Work out the finished part from the listing and answer in its coordinate system (mm). Face numbers are marked on the shaded views. A direction names the side the tool comes from. Give positions to 0.01 mm unless a question says otherwise; leave off trailing zeros. Write each loop counter-clockwise with the first axis right and the second up, starting at its lowest first coordinate (ties: lowest second). Pieces come first, ordered by that corner, then holes. Notation, with made-up numbers: (55, -29.5) -> (110, -29.5) arc R16 cw to (110, -14.5) -> close; hole circle Ø11 at (66.5, 50.25). An arc over 180 degrees is marked (long way). Use a Markdown table: item, result. Add a question column.
Q1. Consider line 1 (Y direction, x = 53.5, z = 1.1); line 2 (Z direction, x = 38.7, y = 46.25); line 3 (X direction, y = 49.5, z = 0.5). Determine where each line is inside the solid, lowest interval first.
Q2. Section C-C, the plane x = 38.7 is taken. Give the vertices of the cut face in (y, z), plus the area to 3 significant figures.
Q3. Section A-A, the plane y = 46 is taken. Give the vertices of the cut face in (x, z).
Q4. Section B-B, the plane z = 8.6 is taken. Give the vertices of the cut face in (x, y), plus the area to 4 significant figures.
Q5. For a pull along X with two mould halves and no side action, classify the marked faces 1, 2 and 3 as pulls with the +X half, pulls with the -X half, needs draft (parallel to the pull), parting line crosses it, or undercut.
Q6. Section D-D, the plane y = 42.5 is taken. State how many separate pieces and enclosed holes the cut face has, plus the area to 3 significant figures.
Q7. For the marked faces 4, 5, 6 and 7, determine the directions among +Z, -Z, +X, -X, +Y, -Y from which every point of the face is accessible in a straight line to the end or side of a thin tool.
Q8. Each of these flat-tipped pins is pushed along its axis until it touches: pin 1 Ø5 at (x, z) = (39.5, 11) entering from +Y; pin 2 Ø1 at (x, z) = (25, 16.5) entering from +Y; pin 3 Ø4 at (x, z) = (33.5, 9) entering from -Y; pin 4 Ø1 at (x, z) = (31.5, 10.5) entering from -Y. Where does it stop, or does it pass through?
from build123d import *

# Parameters (mm, degrees)
SKETCH_1_R          = 4.01
EXTRUDE_1_DEPTH     = 17.2
SKETCH_2_W          = 16.2
SKETCH_2_H          = 7.2
CUT_EXTRUDE_1_DEPTH = 18
SKETCH_4_W          = 2
SKETCH_4_H          = 20
EXTRUDE_2_DEPTH     = 5
SKETCH_3_R          = 1.6
CUT_EXTRUDE_2_DEPTH = 5
CUT_EXTRUDE_START   = -5
SKETCH_5_R          = 3
CUT_EXTRUDE_3_DEPTH = 12
EXTRUDE_7_DEPTH     = 5
SKETCH_7_R          = 5.25
CUT_EXTRUDE_8_DEPTH = 4
CUT_EXTRUDE_9_REACH = 20
SKETCH_8_R          = 2.6


with BuildPart() as part:
    # ｽｹｯﾁ1 → ﾎﾞｽ - 押し出し1 (new body)
    with BuildSketch(Plane.XY):
        with BuildLine():
            Line((24, 53), (51.7, 53))
            Line((51.7, 53), (51.7, 56))
            Line((51.7, 56), (56.7, 56))
            Line((56.7, 56), (56.7, 36))
            Line((56.7, 36), (51.7, 36))
            Line((51.7, 36), (51.7, 39))
            Line((51.7, 39), (24, 39))
            ThreePointArc((24, 39), (17, 46), (24, 53))
        make_face()
        with Locations((24, 46)):
            Circle(SKETCH_1_R, mode=Mode.SUBTRACT)
    extrude(amount=EXTRUDE_1_DEPTH)

    # ｽｹｯﾁ2 → ｶｯﾄ - 押し出し1 (cut, through all)
    with BuildSketch(Plane(origin=(0, 53, 0), x_dir=(1, 0, 0), z_dir=(0, 1, 0))):
        with Locations((25.1, -8.6)):
            Rectangle(SKETCH_2_W, SKETCH_2_H)
    extrude(amount=-CUT_EXTRUDE_1_DEPTH, mode=Mode.SUBTRACT)

    # ｽｹｯﾁ4 → ﾎﾞｽ - 押し出し2 (add)
    with BuildSketch(Plane(origin=(56.7, 0, 0), x_dir=(0, 0, -1), z_dir=(1, 0, 0))):
        with Locations((-18.2, 46)):
            Rectangle(SKETCH_4_W, SKETCH_4_H)
        with Locations((1, 46)):
            Rectangle(SKETCH_4_W, SKETCH_4_H)
    extrude(amount=-EXTRUDE_2_DEPTH)

    # ｽｹｯﾁ3 → ｶｯﾄ - 押し出し2 (cut)
    with BuildSketch(Plane(origin=(56.7, 0, 0), x_dir=(0, 0, -1), z_dir=(1, 0, 0))):
        with Locations((-16.1, 51.592630867)):
            Circle(SKETCH_3_R)
        with Locations((-1.1, 51.592630867)):
            Circle(SKETCH_3_R)
        with Locations((-16.1, 41.592630867)):
            Circle(SKETCH_3_R)
        with Locations((-1.1, 41.592630867)):
            Circle(SKETCH_3_R)
    extrude(amount=-CUT_EXTRUDE_2_DEPTH, mode=Mode.SUBTRACT)

    # ｽｹｯﾁ5 → ｶｯﾄ - 押し出し3 (cut)
    with BuildSketch(Plane(origin=(56.7, 0, 0), x_dir=(0, 0, -1), z_dir=(1, 0, 0)).offset(CUT_EXTRUDE_START)):
        with Locations((-16.1, 51.592630867)):
            Circle(SKETCH_5_R)
        with Locations((-16.1, 41.592630867)):
            Circle(SKETCH_5_R)
        with Locations((-1.1, 51.592630867)):
            Circle(SKETCH_5_R)
        with Locations((-1.1, 41.592630867)):
            Circle(SKETCH_5_R)
    extrude(amount=-CUT_EXTRUDE_3_DEPTH, mode=Mode.SUBTRACT)

    # ｽｹｯﾁ6 → ﾎﾞｽ - 押し出し7 (add)
    with BuildSketch(Plane(origin=(0, 53, 0), x_dir=(1, 0, 0), z_dir=(0, 1, 0))):
        Polygon((33.2, -3.35), (33.2, -13.85), (38.249508532, -16.030014583), (45.7, -11.225178721), (45.7, -5.974821279), (38.249508532, -1.169985417), align=None)
    extrude(amount=EXTRUDE_7_DEPTH)

    # ｽｹｯﾁ7 → ｶｯﾄ - 押し出し8 (cut)
    with BuildSketch(Plane(origin=(0, 58, 0), x_dir=(1, 0, 0), z_dir=(0, 1, 0))):
        with Locations((38.7, -8.6)):
            Circle(SKETCH_7_R)
    extrude(amount=-CUT_EXTRUDE_8_DEPTH, mode=Mode.SUBTRACT)

    # ｽｹｯﾁ8 → ｶｯﾄ - 押し出し9 (cut, up to next)
    with BuildSketch(Plane(origin=(0, 54, 0), x_dir=(1, 0, 0), z_dir=(0, 1, 0)), mode=Mode.PRIVATE) as cut_extrude_9_sk1:
        with Locations((38.7, -8.6)):
            Circle(SKETCH_8_R)
    cut_extrude_9_tool1 = extrude(cut_extrude_9_sk1.sketch, amount=-CUT_EXTRUDE_9_REACH, mode=Mode.PRIVATE) & part.part
    add(cut_extrude_9_tool1.solids().sort_by_distance((38.7, 54, 8.6))[0], mode=Mode.SUBTRACT)


solid = part.part
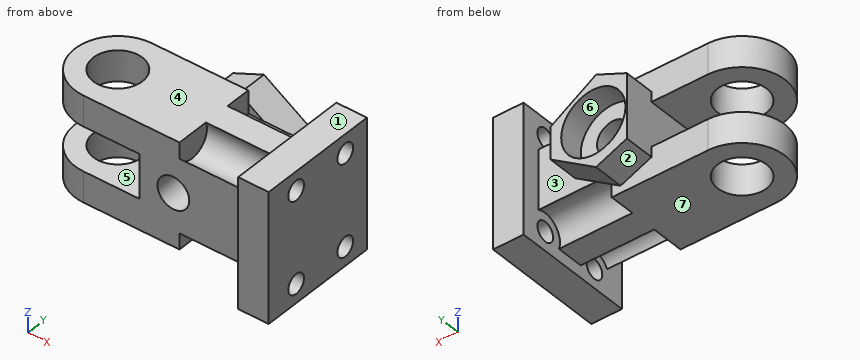
Result set:
| question | item | result |
|---|---|---|
| 1 | line 1 | y = 36 to 39.99, 43.19 to 49.99, 53.19 to 56 |
| 1 | line 2 | z = 0 to 6, 11.2 to 17.2 |
| 1 | line 3 | x = 17.94 to 22.04, 25.96 to 39.7, 51.7 to 56.7 |
| 2 | outline | (39, 0) -> (53, 0) -> (53, 1.46) -> (58, 1.46) -> (58, 3.35) -> (54, 3.35) -> (54, 6) -> (39, 6) -> close; (39, 11.2) -> (54, 11.2) -> (54, 13.85) -> (58, 13.85) -> (58, 15.74) -> (53, 15.74) -> (53, 17.2) -> (39, 17.2) -> close |
| 2 | area | 192 mm2 |
| 3 | outline | (17, 0) -> (19.99, 0) -> (19.99, 5) -> (17, 5) -> close; (17, 12.2) -> (19.99, 12.2) -> (19.99, 17.2) -> (17, 17.2) -> close; (28.01, 0) -> (51.7, 0) -> (51.7, -2) -> (56.7, -2) -> (56.7, 19.2) -> (51.7, 19.2) -> (51.7, 17.2) -> (28.01, 17.2) -> (28.01, 12.2) -> (33.2, 12.2) -> (33.2, 5) -> (28.01, 5) -> close; hole circle Ø5.2 at (38.7, 8.6) |
| 4 | outline | (33.2, 39) -> (36.1, 39) -> (36.1, 54) -> (33.45, 54) -> (33.45, 58) -> (33.2, 58) -> close; (41.3, 39) -> (51.7, 39) -> (51.7, 36) -> (56.7, 36) -> (56.7, 56) -> (51.7, 56) -> (51.7, 53) -> (45.7, 53) -> (45.7, 58) -> (43.95, 58) -> (43.95, 54) -> (41.3, 54) -> close |
| 4 | area | 301.5 mm2 |
| 5 | face 1 | needs draft |
| 5 | face 2 | pulls with the -X half |
| 5 | face 3 | undercut |
| 6 | separate pieces | 5 |
| 6 | enclosed holes | 1 |
| 6 | area | 395 mm2 |
| 7 | face 4 | +Z, -X, +Y, -Y |
| 7 | face 5 | -X, +Y, -Y |
| 7 | face 6 | +Y |
| 7 | face 7 | -Z, -X, +Y, -Y |
| 8 | pin 1 | stops at y = 54 |
| 8 | pin 2 | stops at y = 53 |
| 8 | pin 3 | stops at y = 39 |
| 8 | pin 4 | passes through |
